Can you work these out from the drawing? Everything is in mm from the part's minimum corner. Round coordinates to 2 decimals unless told otherwise and drop trailing zeros. Order: outer loops, then holes, each group sorted by start corner. A loop starts at its lowest first (then second) coordinate and runs counter-clockwise, first axis right, second up. Notation, with made-up numbers: M 50,31 L 62,31 A25 ccw 62,51 Z; hole C 80,82 d7. An arc over 180 degrees is marked long. Write item = value, one per line. Start each with the question number.
Item 1: Please list where these lines run through material, in increasing order: L1, parallel to X at y = 26, z = 1807; L2, parallel to Y at x = 130, z = 848; L3, parallel to X at y = 33.5, z = 1578.5.
Item 2: I want a section at A-A, the plane z = 1764. List the corners of the cut face in (x, y) for me.
Item 3: I want a section at B-B, the plane y = 6. List the corners of the cut face in (x, z) for me, plus the area to 3 significant figures.
Item 4: I'm going to push flat-ended pins straight in: P1, Ø5, axis at x = 64, y = 17.5, coming from the -Z side; P2, Ø1, axis at y = 8.5, z = 942, coming from the -X side. Where does each tip first touch, or does it pass through?
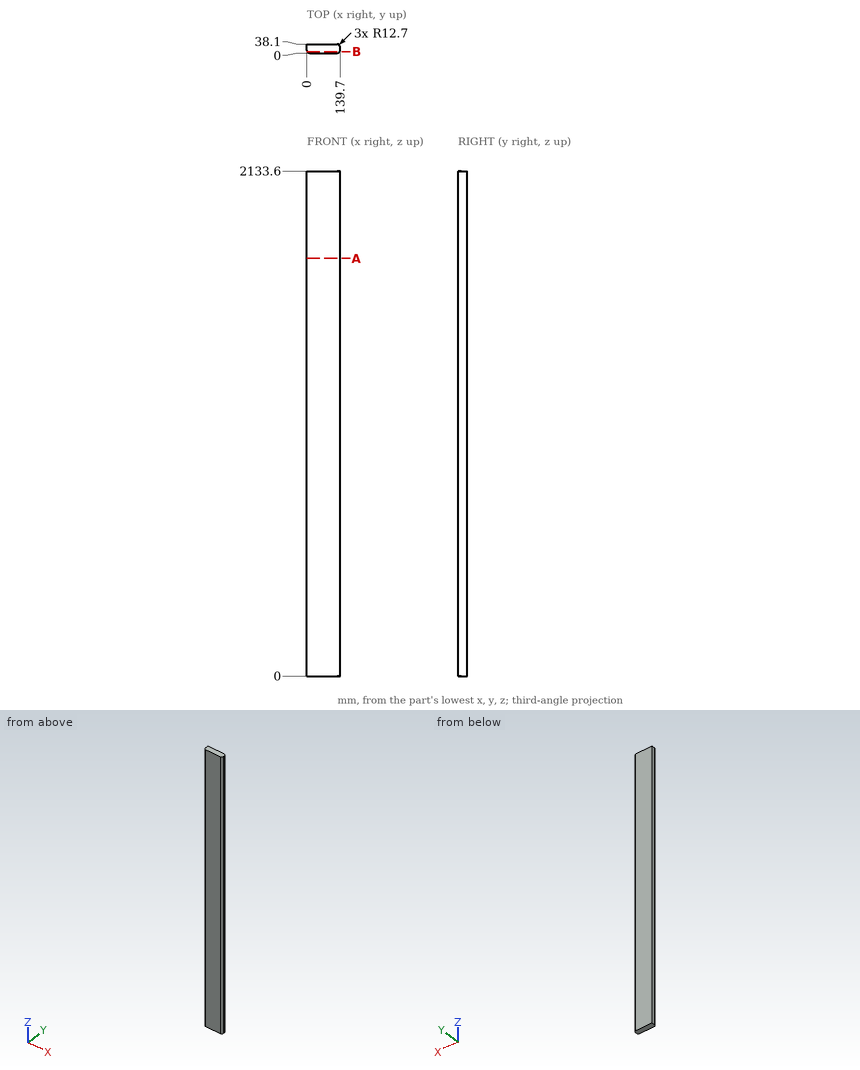
Filled in:
q1.L1 = 0 to 139.69
q1.L2 = 0.36 to 37.74
q1.L3 = 0 to 136.78
q2.outline = M 0,12.7 A12.7 ccw 12.7,0 L 127,0 A12.7 ccw 139.7,12.7 L 139.7,25.4 A12.7 ccw 127,38.1 L 0,38.1 Z
q3.outline = M 1.91,0 L 137.79,0 L 137.79,2133.6 L 1.91,2133.6 Z
q3.area = 290,000 mm^2
q4.P1 = 0
q4.P2 = 0.55
